Read the model definition and answer for the solid it produces. Units are mm, in the model's axes. Face numbers are marked on the shaded views. A direction names the side the tool comes from. Give positions to 0.01 mm unless a question says otherwise; leave off trailing zeros. Order: outer loops, then holes, each group sorted by start corner. A loop starts at its lowest first (then second) coordinate and runs counter-clockwise, first axis right, second up. Notation, with made-up numbers: (48, 55) - (101, 55) arc R15 cw to (101, 60) - close; hole circle Ø6 at (29.25, 36.25). An arc over 180 degrees is marked (long way). Return JSON: item names as keys, results as strings.
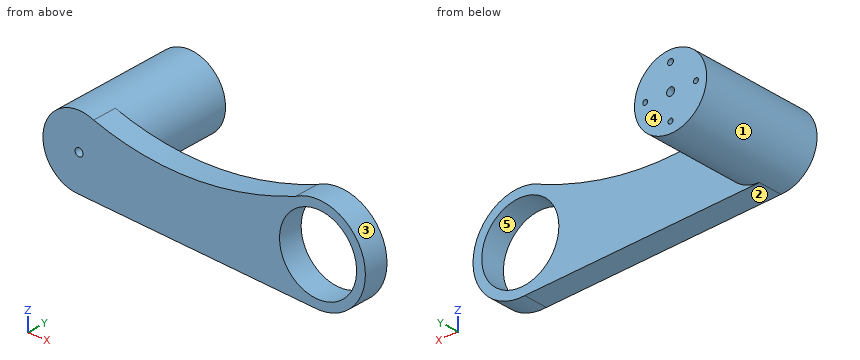
```python
from build123d import *

# Parameters (mm, degrees)
SZKIC1_R                    = 10.3
DODANIE_WYCI_GNI_CIE1_DEPTH = 35.75
OTWORY_USTALAJ_CE_2_5MM2_D  = 2.25
DODANIE_WYCI_GNI_CIE3_START = -7
DODANIE_WYCI_GNI_CIE3_DEPTH = 7
OTWORY_USTALAJ_CE_2_5MM3_D  = 22
SZKIC12_R                   = 0.7
SZKIC12_R_2                 = 0.820346338
WYTNIJ_WYCI_GNI_CIE1_DEPTH  = 7


with BuildPart() as part:
    # Szkic1 → Dodanie-wyciągnięcie1 (new body)
    with BuildSketch(Plane(origin=(0, 0, 0), x_dir=(1, 0, 0), z_dir=(0, 1, 0))):
        with Locations(Location((0, 0, 0), (0, 0, 270))):
            Circle(SZKIC1_R)
    extrude(amount=DODANIE_WYCI_GNI_CIE1_DEPTH)

    # Otwory ustalające Ø2.5mm2 (through all)
    with Locations(Plane.XZ):
        with Locations((0, 0)):
            Hole(OTWORY_USTALAJ_CE_2_5MM2_D / 2)

    # Szkic7 → Dodanie-wyciągnięcie3 (add)
    with BuildSketch(Plane(origin=(0, 35.75, 0), x_dir=(1, 0, 0), z_dir=(0, 1, 0)).offset(DODANIE_WYCI_GNI_CIE3_START)):
        with BuildLine():
            Line((66.943357066, 13.440701035), (0, 10.3))
            ThreePointArc((0, 10.3), (10.077130906, 2.131063748), (4.169904535, -9.418168408))
            add(Edge.make_bspline(
                [(4.169904535, -9.418168408), (22.461776037, -3.24596138), (41.934151815, -4.077243057), (61.820006497, -11.893378905)],
                knots=[0, 0, 0, 0, 1, 1, 1, 1], degree=3))
            ThreePointArc((61.820006497, -11.893378905), (81.439431711, -2.675954354), (66.943357066, 13.440701035))
        make_face()
    extrude(amount=DODANIE_WYCI_GNI_CIE3_DEPTH)

    # Otwory ustalające Ø2.5mm3 (through all)
    with Locations(Plane(origin=(0, 35.75, 0), x_dir=(1, 0, 0), z_dir=(0, 1, 0))):
        with Locations((68.207301561, 0)):
            Hole(OTWORY_USTALAJ_CE_2_5MM3_D / 2)


with BuildPart() as body_2:
    # Lustro1: mirrored copy
    add(part.part.mirror(Plane.ZX))

    # Szkic12 → Wytnij-wyciągnięcie1 (cut)
    with BuildSketch(Plane(origin=(0, 0, 0), x_dir=(1, 0, 0), z_dir=(0, 1, 0))):
        with Locations(Location((0, 7.24, 0), (0, 0, 270))):
            Circle(SZKIC12_R)
        with Locations(Location((0, -7.24, 0), (0, 0, 270))):
            Circle(SZKIC12_R_2)
        with Locations(Location((7.24, 0, 0), (0, 0, 270))):
            Circle(SZKIC12_R)
        with Locations(Location((-7.24, 0, 0), (0, 0, 270))):
            Circle(SZKIC12_R)
    extrude(amount=-WYTNIJ_WYCI_GNI_CIE1_DEPTH, mode=Mode.SUBTRACT)


solid = body_2.part
```
Q1. A cutting plane is placed at C-C (z = -3.5). Write down the section's boundary in (x, y).
Values:
{"outline": "(-9.69, -35.75) - (57.78, -35.75) - (57.78, -28.75) - (9.69, -28.75) - (9.69, 0) - (-9.69, 0) - close; (78.64, -35.75) - (81.25, -35.75) - (81.25, -28.75) - (78.64, -28.75) - close"}
Q2. For the marked faces 1 and 2, determine the directions among +Z, -Z, +X, -X, +Y, -Y from which every point of the face is accessible in a straight line to the end or side of a thin tool.
Values:
{"face 1": "+Y", "face 2": "-Z, -X, +Y, -Y"}
Q3. Determine the mould class of the marked faces 3, 4 and 5 for opening direction X: released by +X, released by -X, zero draft, split by the parting line, or undercut.
Values:
{"face 3": "split by the parting line", "face 4": "zero draft", "face 5": "undercut"}
Q4. A cutting plane is placed at A-A (z = 4.25). Write down the section's boundary in (x, y), and give its area (3 significant figures).
Values:
{"outline": "(-9.38, -35.75) - (58.06, -35.75) - (58.06, -28.75) - (9.38, -28.75) - (9.38, 0) - (-9.38, 0) - close; (78.35, -35.75) - (81.02, -35.75) - (81.02, -28.75) - (78.35, -28.75) - close", "area": "1,030 mm²"}
Q5. Given pin 1 (6 mm diameter, centred on x = 56.5, y = -28, fed in from +Z); pin 2 (13.5 mm diameter, centred on x = 23.5, z = -5.5, fed in from +Y); pin 3 (5 mm diameter, centred on x = 10, y = -15, fed in from -Z), each flat-ended and moving along its own axis, determine where each tip first touches the part or whether it passes through.
Values:
{"pin 1": "stops at z = 10.98", "pin 2": "stops at y = -28.75", "pin 3": "stops at z = -7.06"}
Q6. Consider L1, parallel to Z at x = 0, y = -26.5 (3 decimals); L2, parallel to Y at x = 24, z = -2.5; L3, parallel to Z at x = 0.5, y = -15.5. Determine where each line is inside the solid, lowest interval first.
Values:
{"L1": "z = -10.3 to -1.125, 1.125 to 10.3", "L2": "y = -35.75 to -28.75", "L3": "z = -10.29 to -1.01, 1.01 to 10.29"}
Q7. A cutting plane is placed at B-B (y = -16). Write down the section's boundary in (x, z) (3 decimals).
Values:
{"outline": "circle Ø20.6 at (0, 0); hole circle Ø2.25 at (0, 0)"}
Q8. A cutting plane is placed at D-D (x = -5). Write down the section's boundary in (y, z) (3 decimals).
Values:
{"outline": "(-35.75, -9.005) - (0, -9.005) - (0, 9.005) - (-35.75, 9.005) - close"}
